```python
from build123d import *

# Parameters (mm, degrees)
EXTRUDE1_DEPTH = 0.15239999999999998
FILLET1_R      = 0.13716


with BuildPart() as part:
    # Sketch2 → Extrude1 (new, symmetric)
    with BuildSketch(Plane.XY):
        with BuildLine():
            Line((3.140418046431012, -0.8414724794373154), (3.3857632063084426, -0.9072125168933589))
            ThreePointArc((3.3857632063084426, -0.9072125168933589), (-3.505200000000001, 4.3e-16), (3.3857632063084426, 0.9072125168933589))
            Line((3.3857632063084426, 0.9072125168933589), (2.895072886553593, 0.7757324419812774))
            ThreePointArc((2.895072886553593, 0.7757324419812774), (-2.920866106263664, 0.6721227784267793), (2.2648416082243603, -1.9630843918832563))
            ThreePointArc((2.2648416082243603, -1.9630843918832563), (2.81661020018612, -1.4912562075486206), (3.140418046431012, -0.8414724794373154))
        make_face()
    extrude(amount=EXTRUDE1_DEPTH, both=True)

    # Fillet1
    fillet1_edges = [part.edges().sort_by_distance(p)[0] for p in [
        (-3.5052000000000008, 2.55e-15, 0.15239999999999998),
        (-2.920866106263662, 0.6721227784267882, 0.15239999999999998),
        (-3.5052000000000008, 2.55e-15, -0.15239999999999998),
        (-2.920866106263662, 0.6721227784267882, -0.15239999999999998),
    ]]
    fillet(fillet1_edges, radius=FILLET1_R)


solid = part.part
```
For this review, take the finished solid that the model builds, in its own axes (mm). Round coordinates to 2 decimals unless told otherwise and drop trailing zeros. Write each loop counter-clockwise with the first axis right and the second up, starting at its lowest first coordinate (ties: lowest second). Pieces come first, ordered by that corner, then holes. Notation, with made-up numbers: (56.5, 62) - (89.5, 62) arc R20 cw to (89.5, 68) - close; hole circle Ø11 at (21.5, 48). An arc over 180 degrees is marked (long way). Write each question's results on one line, items separated by ' | '.
Item 1: To check wall thickness, follow line 1 along Y through (x, z) = (0, 0); line 2 along X through (y, z) = (0, 0); line 3 along X through (y, z) = (-1.5, 0.05). State the ranges of each line that lie inside material, in increasing order. Write a range as from..to.
Calculated:
line 1: y = -3.51..-3, 3..3.51 | line 2: x = -3.51..-3 | line 3: x = -3.16..-2.6, 2.81..3.16
Item 2: For pin 1 (2 mm diameter, centred on x = -1.5, y = 1, fed in from +Z), flat-tipped, find the tip position at first contact; note if it passes through.
Calculated:
pin 1: passes through
Item 3: Take a section at C-C on z = 0.1. State the section outline as (x, y) points.
Calculated:
outline: (2.34, -1.92) arc R3.03 cw (long way) to (2.92, 0.78) - (3.36, 0.9) arc R3.48 ccw (long way) to (3.36, -0.9) - (3.14, -0.84) arc R1.82 cw to start
